from build123d import *

# Parameters (mm, degrees)
BASE_FLANGE1_DEPTH = 250
CHAMFER1_SIZE      = 5
CUT_EXTRUDE1_REACH = 263.498
SKETCH3_R          = 2.25
CUT_EXTRUDE2_REACH = 263.498
SKETCH4_R          = 2.25


# Sheet-metal steps are written as plain solids
with BuildPart() as part:
    # Sketch1 → Base-Flange1 (new body)
    with BuildSketch(Plane.XY):
        with BuildLine():
            Line((-16, 37.5), (-4, 37.5))
            ThreePointArc((-4, 37.5), (-1.171572875, 36.328427125), (0, 33.5))
            Line((0, 33.5), (0, -33.5))
            ThreePointArc((0, -33.5), (-1.171572875, -36.328427125), (-4, -37.5))
            Line((-4, -37.5), (-16, -37.5))
            Line((-16, -37.5), (-16, -35.5))
            Line((-16, -35.5), (-4, -35.5))
            ThreePointArc((-4, -35.5), (-2.585786438, -34.914213562), (-2, -33.5))
            Line((-2, -33.5), (-2, 33.5))
            ThreePointArc((-2, 33.5), (-2.585786438, 34.914213562), (-4, 35.5))
            Line((-4, 35.5), (-16, 35.5))
            Line((-16, 35.5), (-16, 37.5))
        make_face()
    extrude(amount=BASE_FLANGE1_DEPTH)

    # Chamfer1
    chamfer1_edges = [part.edges().sort_by_distance(p)[0] for p in [
        (-16, 36.5, 0),
        (-16, -36.5, 0),
        (-16, 36.5, 250),
        (-16, -36.5, 250),
    ]]
    chamfer(chamfer1_edges, length=CHAMFER1_SIZE)

    # Sketch3 → Cut-Extrude1 (cut, up to next)
    with BuildSketch(Plane(origin=(0, 37.5, 0), x_dir=(1, 0, 0), z_dir=(0, 1, 0)), mode=Mode.PRIVATE) as cut_extrude1_sk1:
        with Locations(Location((-10, -62.5, 0), (0, 0, 270))):
            Circle(SKETCH3_R)
    cut_extrude1_tool1 = extrude(cut_extrude1_sk1.sketch, amount=-CUT_EXTRUDE1_REACH, mode=Mode.PRIVATE) & part.part
    # Sketch3 → Cut-Extrude1 (cut, up to next)
    with BuildSketch(Plane(origin=(0, 37.5, 0), x_dir=(1, 0, 0), z_dir=(0, 1, 0)), mode=Mode.PRIVATE) as cut_extrude1_sk2:
        with Locations(Location((-10, -187.5, 0), (0, 0, 180))):
            Circle(SKETCH3_R)
    cut_extrude1_tool2 = extrude(cut_extrude1_sk2.sketch, amount=-CUT_EXTRUDE1_REACH, mode=Mode.PRIVATE) & part.part
    add(cut_extrude1_tool1.solids().sort_by_distance((-10, 37.5, 62.5))[0], mode=Mode.SUBTRACT)
    add(cut_extrude1_tool2.solids().sort_by_distance((-10, 37.5, 187.5))[0], mode=Mode.SUBTRACT)

    # Sketch4 → Cut-Extrude2 (cut, up to next)
    with BuildSketch(Plane.XZ.offset(37.5), mode=Mode.PRIVATE) as cut_extrude2_sk1:
        with Locations(Location((-10, 31.25, 0), (0, 0, 270))):
            Circle(SKETCH4_R)
    cut_extrude2_tool1 = extrude(cut_extrude2_sk1.sketch, amount=-CUT_EXTRUDE2_REACH, mode=Mode.PRIVATE) & part.part
    # Sketch4 → Cut-Extrude2 (cut, up to next)
    with BuildSketch(Plane.XZ.offset(37.5), mode=Mode.PRIVATE) as cut_extrude2_sk2:
        with Locations(Location((-10, 93.75, 0), (0, 0, 270))):
            Circle(SKETCH4_R)
    cut_extrude2_tool2 = extrude(cut_extrude2_sk2.sketch, amount=-CUT_EXTRUDE2_REACH, mode=Mode.PRIVATE) & part.part
    # Sketch4 → Cut-Extrude2 (cut, up to next)
    with BuildSketch(Plane.XZ.offset(37.5), mode=Mode.PRIVATE) as cut_extrude2_sk3:
        with Locations(Location((-10, 156.25, 0), (0, 0, 270))):
            Circle(SKETCH4_R)
    cut_extrude2_tool3 = extrude(cut_extrude2_sk3.sketch, amount=-CUT_EXTRUDE2_REACH, mode=Mode.PRIVATE) & part.part
    # Sketch4 → Cut-Extrude2 (cut, up to next)
    with BuildSketch(Plane.XZ.offset(37.5), mode=Mode.PRIVATE) as cut_extrude2_sk4:
        with Locations(Location((-10, 218.75, 0), (0, 0, 270))):
            Circle(SKETCH4_R)
    cut_extrude2_tool4 = extrude(cut_extrude2_sk4.sketch, amount=-CUT_EXTRUDE2_REACH, mode=Mode.PRIVATE) & part.part
    add(cut_extrude2_tool1.solids().sort_by_distance((-10, -37.5, 31.25))[0], mode=Mode.SUBTRACT)
    add(cut_extrude2_tool2.solids().sort_by_distance((-10, -37.5, 93.75))[0], mode=Mode.SUBTRACT)
    add(cut_extrude2_tool3.solids().sort_by_distance((-10, -37.5, 156.25))[0], mode=Mode.SUBTRACT)
    add(cut_extrude2_tool4.solids().sort_by_distance((-10, -37.5, 218.75))[0], mode=Mode.SUBTRACT)


solid = part.part
Geometry: final body of the model. Coordinates: model frame, mm. A direction names the side the tool comes from. Coordinates: 2 decimals unless noted, no trailing zeros. Loops run counter-clockwise (first coordinate to the right, second up) from the corner with the lowest first, then second, coordinate; pieces in that order, holes last. Notation, with made-up numbers: (-6.75, -7) - (29.25, -7) arc R21 ccw to (29.25, 13) - close; hole circle Ø5 at (-27.5, -40). An arc over 180 degrees is marked (long way). One line per question, with ' | ' between items. Start each with the question number.
(1) Cut plane B-B on y = -12. Output: boundary loops of the cut face in (x, z), and give its area (3 significant figures).
(2) First-contact query: pin 1 (20 mm diameter, centred on y = 5.5, z = 157, fed in from -X). Flat tip, straight axial feed; report the tip coordinate or a pass-through.
(3) Reachability of faces 5 (the flat face through (-2, 0, 123)), 6 (the cylindrical face through (-9.512, 36.514, 185.304)), 7 (the cylindrical face through (-9.324, -36.514, 91.604)) from +Z, -Z, +X, -X, +Y, -Y: full face, straight path, thin tool, end or side. Return the list, or none.
(4) Cut plane A-A on z = 31.25. Output: boundary loops of the cut face in (x, y).
(5) Ray query, L1, parallel to Y at x = -8.5, z = 234; L2, parallel to X at y = 21, z = 65.5; L3, parallel to Y at x = -3.5, z = 192.5. Return the intervals inside material, ascending. Write a range as from..to.
(6) Draft query along Y for faces 1 (the flat face through (-10, 37.5, 123)), 2 (the flat face through (-13, 36, 248)), 3 (the flat face through (-10, -37.5, 123)), 4 (the flat face through (-10, -35.5, 123)). Return one class per face: +Y half, -Y half, draft (parallel to the pull), parting line (faces both ways), or undercut.
Here are the results:
1) outline: (-2, 0) - (0, 0) - (0, 250) - (-2, 250) - close | area: 500 mm²
2) pin 1: x = -2
3) face 5: +Z, -Z, -X | face 6: +Y | face 7: -Y
4) outline: (-16, -37.5) - (-12.25, -37.5) - (-12.25, -35.5) - (-16, -35.5) - close; (-16, 35.5) - (-4, 35.5) arc R2 cw to (-2, 33.5) - (-2, -33.5) arc R2 cw to (-4, -35.5) - (-7.75, -35.5) - (-7.75, -37.5) - (-4, -37.5) arc R4 ccw to (0, -33.5) - (0, 33.5) arc R4 ccw to (-4, 37.5) - (-16, 37.5) - close
5) L1: -37.5..-35.5, 35.5..37.5 | L2: -2..0 | L3: -37.47..-35.44, 35.44..37.47
6) face 1: +Y half | face 2: draft | face 3: -Y half | face 4: undercut
